Here's how the part is built. I have some questions about the finished solid (model axes, mm). Face numbers are marked on the shaded views. A direction names the side the tool comes from. Round coordinates to 2 decimals unless told otherwise and drop trailing zeros. Order: outer loops, then holes, each group sorted by start corner. A loop starts at its lowest first (then second) coordinate and runs counter-clockwise, first axis right, second up.
```python
from build123d import *

# Parameters (mm, degrees)
SKETCH_1_R      = 1.5
EXTRUDE_1_DEPTH = 4


with BuildPart() as part:
    # 草图1 → 凸台-拉伸1 (new body)
    with BuildSketch(Plane.XY):
        with BuildLine():
            Line((-8.883361298, 38.430372232), (-10.42356995, 28.043950456))
            ThreePointArc((-10.42356995, 28.043950456), (-10.775128008, 27.17392517), (-11.484802252, 26.560003729))
            ThreePointArc((-11.484802252, 26.560003729), (-13.893149851, 24.653752275), (-15.405733358, 21.980547476))
            ThreePointArc((-15.405733358, 21.980547476), (-20.465380085, 19.450724806), (-22.995202754, 24.510371532))
            Line((-22.995202754, 24.510371532), (-18.451197233, 38.142383115))
            ThreePointArc((-18.451197233, 38.142383115), (-18.348830032, 38.742204214), (-18.431570381, 39.345046174))
            Line((-18.431570381, 39.345046174), (-22.233001172, 52.125165651))
            ThreePointArc((-22.233001172, 52.125165651), (-22.31526172, 52.64074939), (-22.261276417, 53.160055635))
            Line((-22.261276417, 53.160055635), (-18.372774426, 69.438220218))
            ThreePointArc((-18.372774426, 69.438220218), (-18.096529541, 70.075517478), (-17.618975762, 70.579899696))
            Line((-17.618975762, 70.579899696), (-6.150614111, 79.086205979))
            ThreePointArc((-6.150614111, 79.086205979), (-5.627950875, 79.131232586), (-5.352746621, 78.684615443))
            Line((-5.352746621, 78.684615443), (-5.352746621, 75.677999772))
            ThreePointArc((-5.352746621, 75.677999772), (-14.888864346, 58.677248629), (-9.31952103, 39.997165768))
            ThreePointArc((-9.31952103, 39.997165768), (-8.934989705, 39.260105305), (-8.883361298, 38.430372232))
        make_face()
        with Locations((-19.200468056, 23.245459504)):
            Circle(SKETCH_1_R, mode=Mode.SUBTRACT)
        with Locations((-14.200468056, 38.245459504)):
            Circle(SKETCH_1_R, mode=Mode.SUBTRACT)
    extrude(amount=EXTRUDE_1_DEPTH)


solid = part.part
```
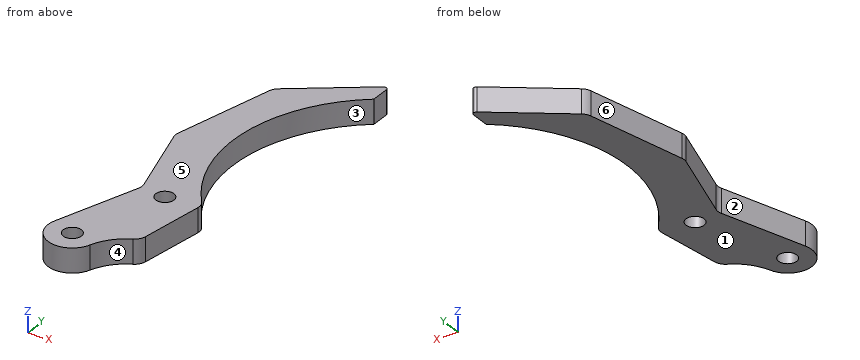
1) We'd pull the mould along Y, two halves only. Please class the marked faces 3, 4, 5 and 6: +Y half, -Y half, draft (parallel to the pull), parting line (faces both ways), or undercut.
2) For the marked faces 1 and 2, which set-ups out of +Z, -Z, +X, -X, +Y, -Y let a thin tool reach every point of the face, with its end or its side?
3) If we section it at B-B (z = 1.95): Write out the boundary of the cut face in (x, y), plus the area to 3 significant figures.
4) I need wall thicknesses on line 1 (Y direction, x = -11, z = 3.65); line 2 (X direction, y = 33.5, z = 3.45); line 3 (X direction, y = 35.5, z = 1.5). Which ranges of each line are inside material? Lowest first, please.
5) If we section it at C-C (y = 68.5): Write out the boundary of the cut face in (x, z), plus the area to 3 significant figures.
6) If we section it at D-D (x = -7.5): Write out the boundary of the cut face in (y, z), plus the area to 3 significant figures.
7) If we section it at A-A (x = -21.25): Write out the boundary of the cut face in (y, z), plus the area to 3 significant figures.
8) I'm going to push a flat-ended pin straight in: pin 1 (4 mm diameter, centred on x = -13.5, y = 55.5, fed in from +Z). Where does the tip first touch, or does it pass through?
Solutions:
1. face 3: undercut
1. face 4: -Y half
1. face 5: draft
1. face 6: +Y half
2. face 1: -Z, +X, -X, +Y, -Y
2. face 2: +Z, -Z, -X
3. outline: (-23, 24.51) arc R4 ccw to (-15.41, 21.98) arc R8 cw to (-11.48, 26.56) arc R2 ccw to (-10.42, 28.04) - (-8.88, 38.43) arc R2 ccw to (-9.32, 40) arc R25 cw to (-5.35, 75.68) - (-5.35, 78.68) arc R0.5 ccw to (-6.15, 79.09) - (-17.62, 70.58) arc R2 ccw to (-18.37, 69.44) - (-22.26, 53.16) arc R2 ccw to (-22.23, 52.13) - (-18.43, 39.35) arc R2 cw to (-18.45, 38.14) - close; hole circle Ø3 at (-19.2, 23.25); hole circle Ø3 at (-14.2, 38.25)
3. area: 437 mm2
4. line 1: y = 26.91 to 42.29, 69.54 to 75.49
4. line 2: x = -20 to -9.61
4. line 3: x = -19.33 to -9.32
5. outline: (-18.6, 0) - (-11.64, 0) - (-11.64, 4) - (-18.6, 4) - close
5. area: 27.8 mm2
6. outline: (73.81, 0) - (78.09, 0) - (78.09, 4) - (73.81, 4) - close
6. area: 17.1 mm2
7. outline: (19.81, 0) - (29.75, 0) - (29.75, 4) - (19.81, 4) - close; (48.82, 0) - (57.39, 0) - (57.39, 4) - (48.82, 4) - close
7. area: 74.0 mm2
8. pin 1: stops at z = 4
